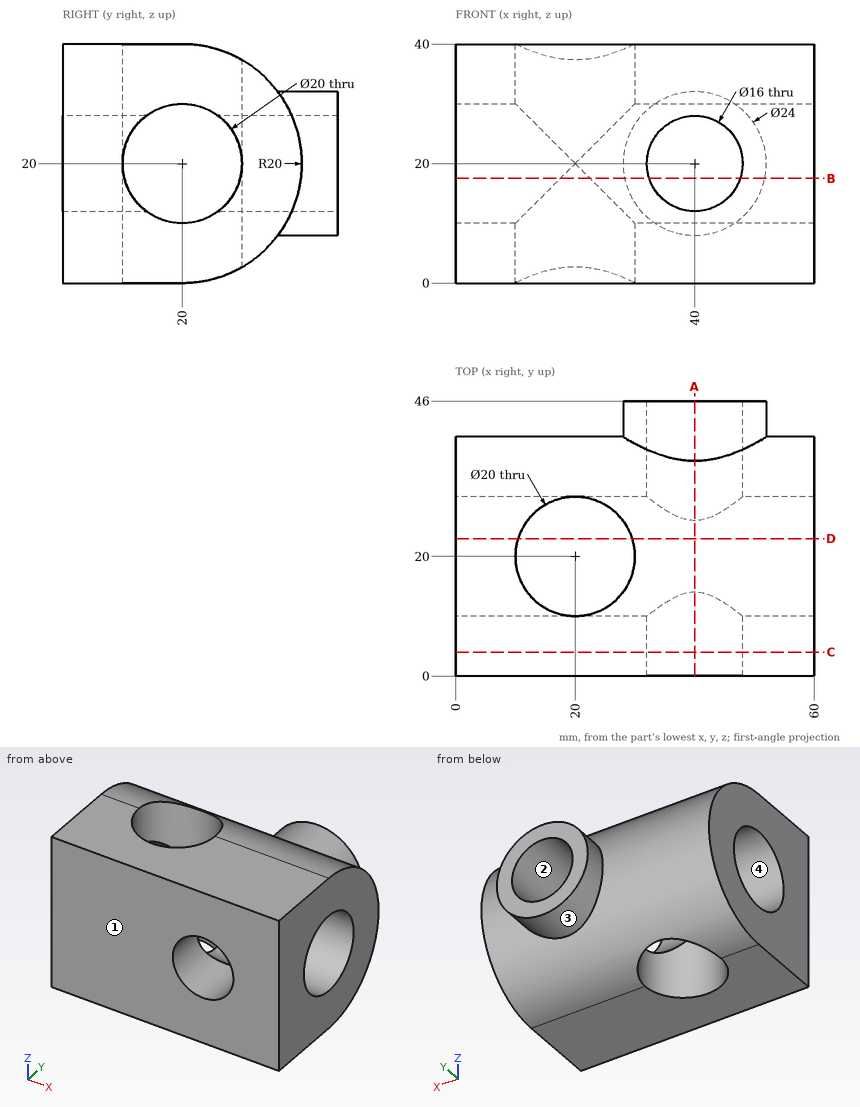
Could you check a few things on this drawing? It's one solid part, dimensions in mm from its lowest x, y, z. Coordinates: 2 decimals unless noted, no trailing zeros. Order: outer loops, then holes, each group sorted by start corner. A loop starts at its lowest first (then second) coordinate and runs counter-clockwise, first axis right, second up. Notation, with made-up numbers: M 27.5,-15 L 86.5,-15 A24 ccw 86.5,17 Z; hole C 51,-40 d4. An arc over 180 degrees is marked long. Use a Markdown table: item, result. Add a question column.
Q1. I want a section at C-C on y = 4. List the corners of the cut face in (x, z) for me.
Q2. I want a section at D-D on y = 23. List the corners of the cut face in (x, z) for me, then the cut area to 3 significant figures.
Q3. I want a section at B-B on z = 17.5. List the corners of the cut face in (x, y) for me.
Q4. I'm going to push flat-ended pins straight in: pin 1 (1 mm diameter, centred on x = 30, y = 31.5, fed in from -Z); pin 2 (4 mm diameter, centred on x = 13, z = 29.5, fed in from +Y); pin 3 (9.5 mm diameter, centred on x = 40, z = 20, fed in from -Y); pin 4 (12 mm diameter, centred on x = 42, z = 13.5, fed in from -Y). Where does each tip first touch, or does it pass through?
Q5. If I drill on L1, parallel to Y at x = 48, z = 12; L2, parallel to Z at x = 43, y = 14; L3, parallel to Y at x = 15.5, z = 20, over which ranges is the centre line in solid material (lowest first)?
Q6. We'd pull the mould along Z, two halves only. Please class the marked faces 1, 2, 3 and 4: pulls with the +Z half, pulls with the -Z half, needs draft (parallel to the pull), parting line crosses it, or undercut.
Q7. I want a section at A-A on x = 40. List the corners of the cut face in (y, z) for me.
Checked values:
| question | item | result |
|---|---|---|
| 1 | outline | M 0,0 L 60,0 L 60,40 L 0,40 Z; hole C 40,20 d16 |
| 2 | outline | M 0,0.23 L 10.46,0.23 L 10.46,10.46 L 0,10.46 Z; M 0,29.54 L 10.46,29.54 L 10.46,39.77 L 0,39.77 Z; M 29.54,0.23 L 60,0.23 L 60,10.46 L 29.54,10.46 Z; M 29.54,29.54 L 60,29.54 L 60,39.77 L 29.54,39.77 Z |
| 2 | area | 838 mm² |
| 3 | outline | M 0,0 L 32.4,0 L 32.4,10.32 L 22.5,10.32 A10 cw 17.5,10.32 L 0,10.32 Z; M 0,29.68 L 17.5,29.68 A10 cw 22.5,29.68 L 32.4,29.68 L 32.4,46 L 28.26,46 L 28.26,39.84 L 0,39.84 Z; M 47.6,0 L 60,0 L 60,10.32 L 47.6,10.32 Z; M 47.6,29.68 L 60,29.68 L 60,39.84 L 51.74,39.84 L 51.74,46 L 47.6,46 Z |
| 4 | pin 1 | z = 3.3 |
| 4 | pin 2 | y = 38.54 |
| 4 | pin 3 | through |
| 4 | pin 4 | y = 0 |
| 5 | L1 | 0 to 14, 26 to 46 |
| 5 | L2 | 0 to 12, 28 to 40 |
| 5 | L3 | 0 to 10, 30 to 40 |
| 6 | face 1 | needs draft |
| 6 | face 2 | undercut |
| 6 | face 3 | parting line crosses it |
| 6 | face 4 | undercut |
| 7 | outline | M 0,0 L 20,0 A20 ccw 36,8 L 46,8 L 46,12 L 26,12 A10 cw 14,12 L 0,12 Z; M 0,28 L 14,28 A10 cw 26,28 L 46,28 L 46,32 L 36,32 A20 ccw 20,40 L 0,40 Z |
